```python
from build123d import *

# Parameters (mm, degrees)
SKETCH_1_R               = 50
EXTRUDE_1_DEPTH          = 80
CUT_EXTRUDE_START        = -40
CUT_EXTRUDE_1_DEPTH      = 40
FILLET_1_R               = 5
CUT_EXTRUDE_2_DEPTH      = 107.770782689
CUT_EXTRUDE_2_DEPTH_BACK = 107.770782689
SKETCH_3_R               = 12.5
CHAMFER_1_SIZE           = 3
CUT_EXTRUDE_3_DEPTH      = 107.770782689
CUT_EXTRUDE_3_DEPTH_BACK = 107.770782689
SKETCH_4_R               = 10


with BuildPart() as part:
    # Эскиз1 → Бобышка-Вытянуть1 (new body)
    with BuildSketch(Plane.XY):
        Circle(SKETCH_1_R)
    extrude(amount=EXTRUDE_1_DEPTH)

    # Эскиз2 → Вырез-Вытянуть1 (cut)
    with BuildSketch(Plane.XY.offset(80).offset(CUT_EXTRUDE_START)):
        with BuildLine():
            Line((-22.5, 44.651427749), (-22.5, -44.651427749))
            ThreePointArc((-22.5, -44.651427749), (-50, 0), (-22.5, 44.651427749))
        make_face()
        with BuildLine():
            Line((22.5, 44.651427749), (22.5, -44.651427749))
            ThreePointArc((22.5, -44.651427749), (50, 0), (22.5, 44.651427749))
        make_face()
    extrude(amount=CUT_EXTRUDE_1_DEPTH, mode=Mode.SUBTRACT)

    # Скругление1
    fillet_1_edges = [part.edges().sort_by_distance(p)[0] for p in [
        (22.5, 0, 40),
        (-22.5, 0, 40),
    ]]
    fillet(fillet_1_edges, radius=FILLET_1_R)

    # Эскиз3 → Вырез-Вытянуть2 (cut, two sides: drawn at the far end of the back side and taken through both)
    with BuildSketch(Plane(origin=(0, 0, 0), x_dir=(0, 0, -1), z_dir=(1, 0, 0)).offset(-CUT_EXTRUDE_2_DEPTH_BACK)):
        with Locations(Location((-55, 0, 0), (0, 0, 36.869897646))):
            Circle(SKETCH_3_R)
    extrude(amount=CUT_EXTRUDE_2_DEPTH + CUT_EXTRUDE_2_DEPTH_BACK, mode=Mode.SUBTRACT)

    # Фаска1
    chamfer_1_edges = [part.edges().sort_by_distance(p)[0] for p in [
        (-50, 0, 0),
    ]]
    chamfer(chamfer_1_edges, length=CHAMFER_1_SIZE)

    # Эскиз4 → Вырез-Вытянуть3 (cut, two sides: drawn at the far end of the back side and taken through both)
    with BuildSketch(Plane(origin=(0, 0, 0), x_dir=(0, 0, -1), z_dir=(1, 0, 0)).offset(-CUT_EXTRUDE_3_DEPTH_BACK)):
        with Locations((-15, 0)):
            Circle(SKETCH_4_R)
    extrude(amount=CUT_EXTRUDE_3_DEPTH + CUT_EXTRUDE_3_DEPTH_BACK, mode=Mode.SUBTRACT)


solid = part.part
```
Could you check a few things on this model? Use its own coordinates, in mm. A direction names the side the tool comes from. Coordinates: 2 decimals unless noted, no trailing zeros. Write each loop counter-clockwise with the first axis right and the second up, starting at its lowest first coordinate (ties: lowest second). Pieces come first, ordered by that corner, then holes. Notation, with made-up numbers: (-38, -28) -> (18, -28) arc R17 ccw to (18, -24) -> close; hole circle Ø9 at (-27.5, 56.5). An arc over 180 degrees is marked (long way). Write item = value, one per line. Start each with the question number.
(1) I need wall thicknesses on line 1 (Z direction, x = 21, y = 0); line 2 (Z direction, x = 32, y = -30); line 3 (X direction, y = 21.5, z = 71). Which ranges of each line are inside material? Lowest first, please. Write a range as [from, to].
(2) Which directions (+Z, -Z, +X, -X, +Y, -Y) give clear straight access to the entire face, cutting with the end or side of a thin tool? Please do faces 4 (the face through (-6.137, 46.744, 0.146)), 5 (the face through (22.5, 1, 70)), 6 (the face through (-36, 1, 40)).
(3) I want a section at A-A (z = 55). Please give me the cut outline in (x, y).
(4) I want a section at D-D (z = 15). Please give me the cut outline in (x, y), plus the area to 3 significant figures.
(5) I want a section at C-C (x = 0). Please give me the cut outline in (y, z).
(6) We'd pull the mould along Z, two halves only. Please class faces 1 (the face through (-1, 1, 0)), 2 (the face through (24, -0.63, 41.43)), 3 (the face through (-0.7, 3, 5.46)): released by +Z, released by -Z, zero draft, split by the parting line, or undercut.
(7) Will these pins go through, and if not, where does the flat tip stop? pin 1 (2 mm diameter, centred on x = -10.5, z = 59, fed in from -Y); pin 2 (10 mm diameter, centred on x = 31.5, y = -0.5, fed in from +Z); pin 3 (2 mm diameter, centred on y = -37.5, z = 16.5, fed in from +X); pin 4 (12 mm diameter, centred on x = 20.5, y = 27, fed in from -Z).
(8) I want a section at B-B (y = 0). Please give me the cut outline in (x, z), plus the area to 3 significant figures.
Result set:
q1.line_1 = [0, 5], [25, 42.5], [67.5, 80]
q1.line_2 = [0, 40]
q1.line_3 = [-22.5, 22.5]
q2.face_4 = -Z
q2.face_5 = +Z, +X, +Y, -Y
q2.face_6 = +Z, -X, +Y, -Y
q3.outline = (-22.5, -44.65) arc R50 ccw to (22.5, -44.65) -> (22.5, -12.5) -> (-22.5, -12.5) -> close; (-22.5, 12.5) -> (22.5, 12.5) -> (22.5, 44.65) arc R50 ccw to (-22.5, 44.65) -> close
q4.outline = (-48.99, -10) arc R50 ccw to (48.99, -10) -> close; (-48.99, 10) -> (48.99, 10) arc R50 ccw to start
q4.area = 5,870 mm2
q5.outline = (-50, 3) -> (-47, 0) -> (47, 0) -> (50, 3) -> (50, 80) -> (-50, 80) -> close; hole circle Ø25 at (0, 55); hole circle Ø20 at (0, 15)
q6.face_1 = released by -Z
q6.face_2 = released by +Z
q6.face_3 = undercut
q7.pin_1 = -49.09
q7.pin_2 = 40.1
q7.pin_3 = 34.17
q7.pin_4 = 0
q8.outline = (-50, 3) -> (-47, 0) -> (47, 0) -> (50, 3) -> (50, 5) -> (-50, 5) -> close; (-50, 25) -> (50, 25) -> (50, 40) -> (27.5, 40) arc R5 cw to (23.17, 42.5) -> (-23.17, 42.5) arc R5 cw to (-27.5, 40) -> (-50, 40) -> close; (-22.5, 67.5) -> (22.5, 67.5) -> (22.5, 80) -> (-22.5, 80) -> close
q8.area = 2,680 mm2
